The model under review builds one solid part; all positions refer to its coordinate system, in mm. Coordinates: 2 decimals unless noted, no trailing zeros. Write each loop counter-clockwise with the first axis right and the second up, starting at its lowest first coordinate (ties: lowest second). Pieces come first, ordered by that corner, then holes. Notation, with made-up numbers: (61.5, -6) -> (82.5, -6) arc R16 ccw to (82.5, 5) -> close; hole circle Ø1 at (-23, 88). An arc over 180 degrees is marked (long way). Put each result on its own line as item: value. Start each with the question number.
from build123d import *

# Parameters (mm, degrees)
SKETCH_1_W          = 136
SKETCH_1_H          = 40
EXTRUDE_1_DEPTH     = 2
SKETCH_2_R          = 1.525
CUT_EXTRUDE_1_DEPTH = 2
SKETCH_3_R          = 1.525
CUT_EXTRUDE_2_DEPTH = 22
SKETCH_4_W          = 18.5
SKETCH_4_H          = 28
CUT_EXTRUDE_3_DEPTH = 22
EXTRUDE_2_DEPTH     = 2
SKETCH_6_W          = 9.5
SKETCH_6_H          = 28
CUT_EXTRUDE_4_DEPTH = 2
FILLET_1_R          = 2
SKETCH_7_W          = 19
SKETCH_7_H          = 28
CUT_EXTRUDE_5_DEPTH = 2
EXTRUDE_3_DEPTH     = 2
FILLET_2_R          = 2
FILLET_3_R          = 2


with BuildPart() as part:
    # 草图1 → 凸台-拉伸1 (new body)
    with BuildSketch(Plane.XY):
        Rectangle(SKETCH_1_W, SKETCH_1_H)
    extrude(amount=EXTRUDE_1_DEPTH)

    # 草图2 → 切除-拉伸1 (cut)
    with BuildSketch(Plane(origin=(0, 0, 0), x_dir=(-1, 0, 0), z_dir=(0, 0, -1))):
        with Locations((-34, -6.5)):
            Circle(SKETCH_2_R)
        with Locations((-34, -16.5)):
            Circle(SKETCH_2_R)
        with Locations((16, -6.5)):
            Circle(SKETCH_2_R)
        with Locations((16, -16.5)):
            Circle(SKETCH_2_R)
    extrude(amount=-CUT_EXTRUDE_1_DEPTH, mode=Mode.SUBTRACT)

    # 草图3 → 切除-拉伸2 (cut)
    with BuildSketch(Plane(origin=(0, 0, 0), x_dir=(-1, 0, 0), z_dir=(0, 0, -1))):
        with Locations((65, -15)):
            Circle(SKETCH_3_R)
        with Locations((65, 5)):
            Circle(SKETCH_3_R)
        with Locations((-65, 5)):
            Circle(SKETCH_3_R)
        with Locations((-65, -15)):
            Circle(SKETCH_3_R)
    extrude(amount=-CUT_EXTRUDE_2_DEPTH, mode=Mode.SUBTRACT)

    # 草图4 → 切除-拉伸3 (cut)
    with BuildSketch(Plane.XY.offset(2)):
        with Locations((-51.75, 0)):
            Rectangle(SKETCH_4_W, SKETCH_4_H)
        with Locations((-29.25, 0)):
            Rectangle(SKETCH_4_W, SKETCH_4_H)
    extrude(amount=-CUT_EXTRUDE_3_DEPTH, mode=Mode.SUBTRACT)

    # 草图5 → 凸台-拉伸2 (add)
    with BuildSketch(Plane.XY.offset(2)):
        with BuildLine():
            Line((-53.75, 14), (-53.75, -14))
            ThreePointArc((-53.75, -14), (-51.75, -16), (-49.75, -14))
            Line((-49.75, -14), (-49.75, 14))
            ThreePointArc((-49.75, 14), (-51.75, 16), (-53.75, 14))
        make_face()
        with BuildLine():
            Line((-31.25, 14), (-31.25, -14))
            ThreePointArc((-31.25, -14), (-29.25, -16), (-27.25, -14))
            Line((-27.25, -14), (-27.25, 14))
            ThreePointArc((-27.25, 14), (-29.25, 16), (-31.25, 14))
        make_face()
    extrude(amount=-EXTRUDE_2_DEPTH)

    # 草图6 → 切除-拉伸4 (cut)
    with BuildSketch(Plane.XY.offset(2)):
        with Locations((42.75, 0)):
            Rectangle(SKETCH_6_W, SKETCH_6_H)
        with Locations((56.25, 0)):
            Rectangle(SKETCH_6_W, SKETCH_6_H)
    extrude(amount=-CUT_EXTRUDE_4_DEPTH, mode=Mode.SUBTRACT)

    # 圆角1
    fillet_1_edges = [part.edges().sort_by_distance(p)[0] for p in [
        (-53.75, -14, 1),
        (-49.75, -14, 1),
        (-49.75, 14, 1),
        (-53.75, 14, 1),
        (-31.25, -14, 1),
        (-27.25, -14, 1),
        (-27.25, 14, 1),
        (-31.25, 14, 1),
        (47.5, 14, 1),
        (47.5, -14, 1),
        (38, -14, 1),
        (38, 14, 1),
        (51.5, -14, 1),
        (61, -14, 1),
        (61, 14, 1),
        (51.5, 14, 1),
        (-42.5, 14, 1),
        (-42.5, -14, 1),
        (-61, -14, 1),
        (-61, 14, 1),
        (-38.5, 14, 1),
        (-20, 14, 1),
        (-20, -14, 1),
        (-38.5, -14, 1),
    ]]
    fillet(fillet_1_edges, radius=FILLET_1_R)

    # 草图7 → 切除-拉伸5 (cut)
    with BuildSketch(Plane.XY.offset(2)):
        with Locations((-2.5, 0)):
            Rectangle(SKETCH_7_W, SKETCH_7_H)
        with Locations((20.5, 0)):
            Rectangle(SKETCH_7_W, SKETCH_7_H)
    extrude(amount=-CUT_EXTRUDE_5_DEPTH, mode=Mode.SUBTRACT)

    # 草图8 → 凸台-拉伸3 (add)
    with BuildSketch(Plane.XY.offset(2)):
        with BuildLine():
            Line((-4.5, 14), (-4.5, -14))
            ThreePointArc((-4.5, -14), (-2.5, -16), (-0.5, -14))
            Line((-0.5, -14), (-0.5, 14))
            ThreePointArc((-0.5, 14), (-2.5, 16), (-4.5, 14))
        make_face()
        with BuildLine():
            Line((18.5, 14), (18.5, -14))
            ThreePointArc((18.5, -14), (20.5, -16), (22.5, -14))
            Line((22.5, -14), (22.5, 14))
            ThreePointArc((22.5, 14), (20.5, 16), (18.5, 14))
        make_face()
    extrude(amount=-EXTRUDE_3_DEPTH)

    # 圆角2
    fillet_2_edges = [part.edges().sort_by_distance(p)[0] for p in [
        (7, 14, 1),
        (7, -14, 1),
        (-12, -14, 1),
        (-12, 14, 1),
        (11, -14, 1),
        (30, -14, 1),
        (30, 14, 1),
        (11, 14, 1),
        (-4.5, -14, 1),
        (-0.5, -14, 1),
        (-0.5, 14, 1),
        (-4.5, 14, 1),
        (18.5, -14, 1),
        (22.5, -14, 1),
        (22.5, 14, 1),
        (18.5, 14, 1),
    ]]
    fillet(fillet_2_edges, radius=FILLET_2_R)

    # 圆角3
    fillet_3_edges = [part.edges().sort_by_distance(p)[0] for p in [
        (68, -20, 1),
        (-68, -20, 1),
        (-68, 20, 1),
        (68, 20, 1),
    ]]
    fillet(fillet_3_edges, radius=FILLET_3_R)


solid = part.part
1. Wall thickness on line 1 (Y direction, x = -16, z = 1.4) (3 decimals); line 2 (Y direction, x = 65, z = 1.4) (3 decimals); line 3 (Y direction, x = -9, z = 0.95): over which ranges is each line inside the solid? List them lowest first. Write a range as from..to.
2. Consider section B-B on z = 1. State how many separate pieces and enclosed holes the cut face has, then the cut area to 3 significant figures.
3. Insertion check: P1, Ø4, axis at x = -16, y = -16.5, coming from the +Z side. The pin has a flat end and moves straight along its axis. Give the tip position at first contact, or say it passes through.
4. Consider section A-A on x = -16. State the section outline as (y, z) points (3 decimals), then the cut area to 3 significant figures.
5. The part is to be moulded in two halves that separate along Y. For faces 1 (the cylindrical face through (-16.704, -17.853, 0.986)), 2 (the flat face through (-16, 0, 2)), 3 (the cylindrical face through (-66.4, 4.4, 1)), say which applies: released by +Y, released by -Y, zero draft, split by the parting line, or undercut.
Output values:
1. line 1: y = -20..-18.025, -14.975..-8.025, -4.975..20
1. line 2: y = -20..-16.525, -13.475..3.475, 6.525..20
1. line 3: y = -20..-14, 14..20
2. separate pieces: 1
2. enclosed holes: 18
2. area: 3,230 mm^2
3. P1: stops at z = 2
4. outline: (-20, 0) -> (-18.025, 0) -> (-18.025, 2) -> (-20, 2) -> close; (-14.975, 0) -> (-8.025, 0) -> (-8.025, 2) -> (-14.975, 2) -> close; (-4.975, 0) -> (20, 0) -> (20, 2) -> (-4.975, 2) -> close
4. area: 67.8 mm^2
5. face 1: undercut
5. face 2: zero draft
5. face 3: undercut
